```python
from build123d import *

# Parameters (mm, degrees)
SKETCH1_W               = 89.6
SKETCH1_H               = 75
BOSS_EXTRUDE1_DEPTH     = 1.2
SKETCH2_R               = 28.5
CUT_EXTRUDE1_DEPTH      = 1
CUT_EXTRUDE1_DEPTH_BACK = 2.2


with BuildPart() as part:
    # Sketch1 → Boss-Extrude1 (new body)
    with BuildSketch(Plane(origin=(0, 0, 0), x_dir=(1, 0, 0), z_dir=(0, 1, 0))):
        Rectangle(SKETCH1_W, SKETCH1_H)
    extrude(amount=BOSS_EXTRUDE1_DEPTH)

    # Sketch2 → Cut-Extrude1 (cut, two sides)
    with BuildSketch(Plane(origin=(0, 1.2, 0), x_dir=(1, 0, 0), z_dir=(0, 1, 0))) as cut_extrude1_sk:
        with Locations((14.3, -1.1)):
            Circle(SKETCH2_R)
    extrude(amount=CUT_EXTRUDE1_DEPTH, mode=Mode.SUBTRACT)
    extrude(cut_extrude1_sk.sketch, amount=-CUT_EXTRUDE1_DEPTH_BACK, mode=Mode.SUBTRACT)


solid = part.part
```
Here's how the part is built. I have some questions about the finished solid (model axes, mm). Give positions to 0.01 mm unless a question says otherwise; leave off trailing zeros. Write each loop counter-clockwise with the first axis right and the second up, starting at its lowest first coordinate (ties: lowest second). Pieces come first, ordered by that corner, then holes. Notation, with made-up numbers: (8, -32.5) -> (14, -32.5) arc R23 ccw to (14, 3.5) -> close; hole circle Ø2 at (72, 88). An arc over 180 degrees is marked (long way). Use one line per item in the form item = value.
1) Suppose I cut it at B-B (z = 1.1). Please give me the cut outline in (x, y).
Verdict:
outline = (-44.8, 0) -> (-14.2, 0) -> (-14.2, 1.2) -> (-44.8, 1.2) -> close; (42.8, 0) -> (44.8, 0) -> (44.8, 1.2) -> (42.8, 1.2) -> close
2) Suppose I cut it at C-C (y = 0.4). Please give me the cut outline in (x, z), and give its area (3 significant figures).
Verdict:
outline = (-44.8, -37.5) -> (44.8, -37.5) -> (44.8, 37.5) -> (-44.8, 37.5) -> close; hole circle Ø57 at (14.3, 1.1)
area = 4,170 mm2
3) Suppose I cut it at A-A (x = 14.3). Please give me the cut outline in (y, z), and give its area (3 significant figures).
Verdict:
outline = (0, -37.5) -> (1.2, -37.5) -> (1.2, -27.4) -> (0, -27.4) -> close; (0, 29.6) -> (1.2, 29.6) -> (1.2, 37.5) -> (0, 37.5) -> close
area = 21.6 mm2
4) If I drill on L1, parallel to X at y = 0.3, z = 1.1; L2, parallel to Z at x = 15, y = 0.65; L3, parallel to X at y = 1.1, z = -3, over which ranges is the centre line in solid material (lowest first)? Write a range as [from, to].
Verdict:
L1 = [-44.8, -14.2], [42.8, 44.8]
L2 = [-37.5, -27.39], [29.59, 37.5]
L3 = [-44.8, -13.9], [42.5, 44.8]
5) We'd pull the mould along X, two halves only. Please class faces 1 (the face through (-21, 1.2, -1)), 2 (the face through (41.484, 0.608, -7.461)): +X half, -X half, draft (parallel to the pull), parting line (faces both ways), or undercut.
Verdict:
face_1 = draft
face_2 = undercut
